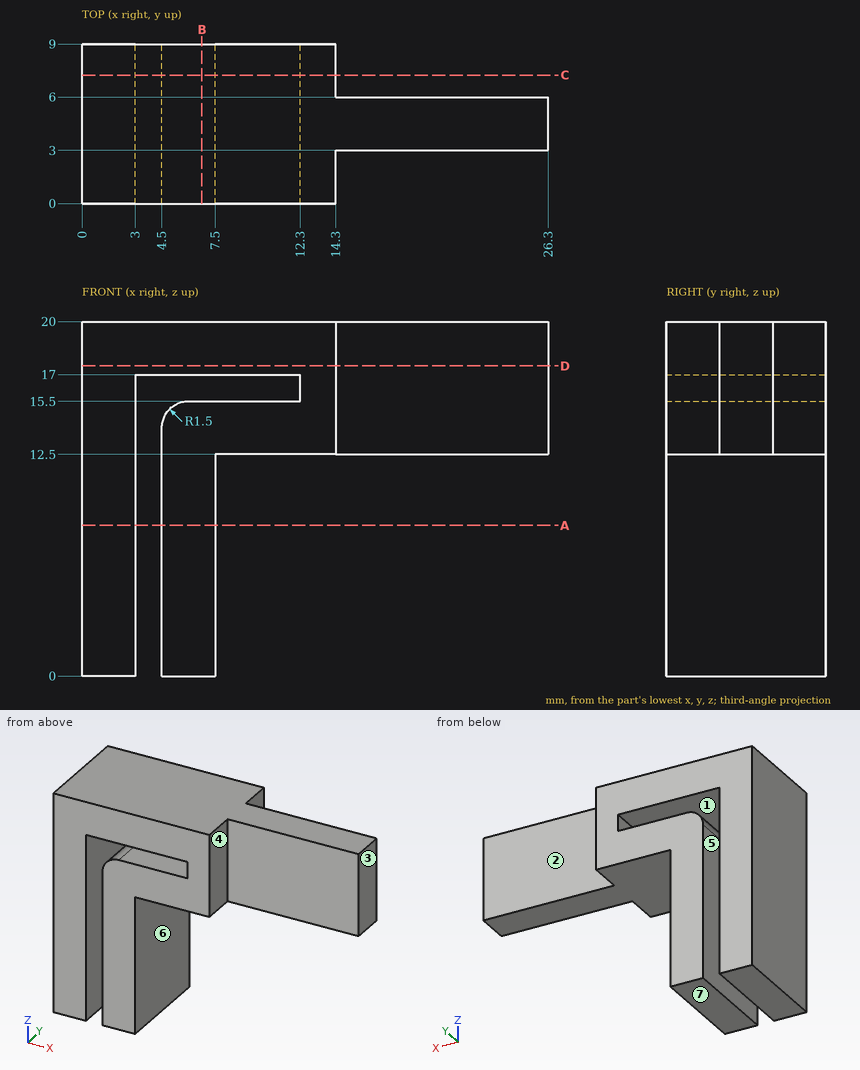
Answer from the drawing. Dimensions are ordinates in mm from the lowest x, y and z of the part. A direction names the side the tool comes from. Coordinates: 2 decimals unless noted, no trailing zeros. Loops run counter-clockwise (first coordinate to the right, second up) from the corner with the lowest first, then second, coordinate; pieces in that order, holes last. Notation, with made-up numbers: (59.5, -12) - (101.5, -12) arc R25 ccw to (101.5, 21) - close; hole circle Ø7 at (-29, 11). An arc over 180 degrees is marked (long way). Use a Markdown table: item, result.
Item 1: Find section B-B, the plane x = 6.75. Determine the outline of the cut face in (y, z), and give its area (4 significant figures).
Evaluation:
| item | result |
|---|---|
| outline | (0, 0) - (9, 0) - (9, 15.5) - (0, 15.5) - close; (0, 17) - (9, 17) - (9, 20) - (0, 20) - close |
| area | 166.5 mm2 |
Item 2: The mould has two halves that part along X. Classify the marked faces 1, 2 and 3: +X half, -X half, draft (parallel to the pull), parting line (faces both ways), or undercut.
Evaluation:
| item | result |
|---|---|
| face 1 | undercut |
| face 2 | draft |
| face 3 | +X half |
Item 3: For the marked faces 4, 5, 6 and 7, determine the directions among +Z, -Z, +X, -X, +Y, -Y from which every point of the face is accessible in a straight line to the end or side of a thin tool.
Evaluation:
| item | result |
|---|---|
| face 4 | +Z, -Z, +X, -Y |
| face 5 | -Z, +Y, -Y |
| face 6 | -Z, +X, +Y, -Y |
| face 7 | -Z, +X, -X, +Y, -Y |
Item 4: Find section D-D, the plane z = 17.5. Determine the outline of the cut face in (x, y).
Evaluation:
| item | result |
|---|---|
| outline | (0, 0) - (14.3, 0) - (14.3, 3) - (26.3, 3) - (26.3, 6) - (14.3, 6) - (14.3, 9) - (0, 9) - close |
Item 5: Find section C-C, the plane y = 7.25. Determine the outline of the cut face in (x, z), and give its area (3 significant figures).
Evaluation:
| item | result |
|---|---|
| outline | (0, 0) - (3, 0) - (3, 17) - (12.3, 17) - (12.3, 15.5) - (6, 15.5) arc R1.5 ccw to (4.5, 14) - (4.5, 0) - (7.5, 0) - (7.5, 12.5) - (14.3, 12.5) - (14.3, 20) - (0, 20) - close |
| area | 163 mm2 |
Item 6: Given pin 1 Ø1.5 at (y, z) = (7.5, 17.5) entering from +X; pin 2 Ø2 at (x, y) = (9.5, 1.5) entering from -Z; pin 3 Ø8 at (x, z) = (23, 16) entering from -Y, each flat-ended and moving along its own axis, determine where each tip first touches the part or whether it passes through.
Evaluation:
| item | result |
|---|---|
| pin 1 | stops at x = 14.3 |
| pin 2 | stops at z = 12.5 |
| pin 3 | stops at y = 3 |
Item 7: Find section A-A, the plane z = 8.5. Determine the outline of the cut face in (x, y), and give its area (3 significant figures).
Evaluation:
| item | result |
|---|---|
| outline | (0, 0) - (3, 0) - (3, 9) - (0, 9) - close; (4.5, 0) - (7.5, 0) - (7.5, 9) - (4.5, 9) - close |
| area | 54.0 mm2 |
Item 8: Consider probe 1 along X at (y, z) = (3.75, 2); probe 2 along Z at (x, y) = (11, 5); probe 3 along Z at (x, y) = (6, 4.25). Determine where each line is inside the solid, lowest interval first. Write a range as from..to.
Evaluation:
| item | result |
|---|---|
| probe 1 | x = 0..3, 4.5..7.5 |
| probe 2 | z = 12.5..15.5, 17..20 |
| probe 3 | z = 0..15.5, 17..20 |
